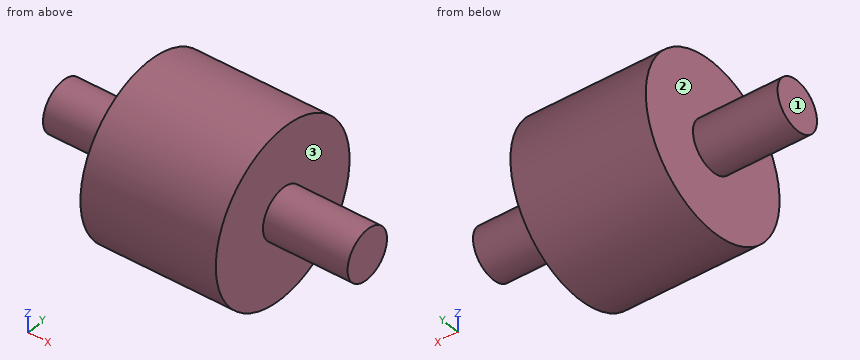
from build123d import *

# Parameters (mm, degrees)
SKETCH1_R                = 25.3837
BOSS_EXTRUDE1_DEPTH      = 40
SKETCH2_R                = 7.485924983
BOSS_EXTRUDE2_DEPTH      = 25
BOSS_EXTRUDE2_DEPTH_BACK = 65


with BuildPart() as part:
    # Sketch1 → Boss-Extrude1 (new body)
    with BuildSketch(Plane(origin=(0, 0, 0), x_dir=(0, 0, -1), z_dir=(1, 0, 0))):
        Circle(SKETCH1_R)
    extrude(amount=BOSS_EXTRUDE1_DEPTH)

    # Sketch2 → Boss-Extrude2 (add, two sides)
    with BuildSketch(Plane.ZY) as boss_extrude2_sk:
        Circle(SKETCH2_R)
    extrude(amount=BOSS_EXTRUDE2_DEPTH)
    extrude(boss_extrude2_sk.sketch, amount=-BOSS_EXTRUDE2_DEPTH_BACK)


solid = part.part
For this review, take the finished solid that the model builds, in its own axes (mm). Face numbers are marked on the shaded views. A direction names the side the tool comes from. Round coordinates to 2 decimals unless told otherwise and drop trailing zeros. Write each loop counter-clockwise with the first axis right and the second up, starting at its lowest first coordinate (ties: lowest second). Pieces come first, ordered by that corner, then holes. Notation, with made-up numbers: (-40, 32.5) - (-15, 32.5) arc R25 cw to (-15, 46.5) - close; hole circle Ø8 at (53, -39). An arc over 180 degrees is marked (long way). Write item = value, one per line. Start each with the question number.
1. Consider section C-C on x = -8. State the section outline as (y, z) points, plus the area to 3 significant figures.
2. For the marked faces 1, 2 and 3, list the 3-axis set-ups (+Z, -Z, +X, -X, +Y, -Y) from which the entire face can be reached by the end or side of a thin tool; tool diameter is ignored.
3. Wall thickness on L1, parallel to X at y = 20, z = 0; L2, parallel to Y at x = 28, z = -16; L3, parallel to Y at x = 36.5, z = 9.5: over which ranges is each line inside the solid? List them lowest first.
4. For pin 1 Ø12 at (y, z) = (-3.5, -19.5) entering from -X; pin 2 Ø1.5 at (x, y) = (11, -12) entering from -Z; pin 3 Ø8 at (x, z) = (16, -13.5) entering from +Y, all flat-tipped, find the tip position at first contact; note any pin that passes through.
5. Consider section A-A on z = 0. State the section outline as (x, y) points.
6. Consider section D-D on x = 22. State the section outline as (y, z) points.
Evaluation:
q1.outline = circle Ø14.97 at (0, 0)
q1.area = 176 mm2
q2.face_1 = +Z, -Z, -X, +Y, -Y
q2.face_2 = -X
q2.face_3 = +X
q3.L1 = 0 to 40
q3.L2 = -19.71 to 19.71
q3.L3 = -23.54 to 23.54
q4.pin_1 = 0
q4.pin_2 = -22.75
q4.pin_3 = 23.54
q5.outline = (-25, -7.49) - (0, -7.49) - (0, -25.38) - (40, -25.38) - (40, -7.49) - (65, -7.49) - (65, 7.49) - (40, 7.49) - (40, 25.38) - (0, 25.38) - (0, 7.49) - (-25, 7.49) - close
q6.outline = circle Ø50.77 at (0, 0)
